Verification items for the finished model (mm, model axes). Face numbers are marked on the shaded views. A direction names the side the tool comes from. Coordinates: 2 decimals unless noted, no trailing zeros. Write each loop counter-clockwise with the first axis right and the second up, starting at its lowest first coordinate (ties: lowest second). Pieces come first, ordered by that corner, then holes. Notation, with made-up numbers: (61.5, -12) -> (68.5, -12) arc R36 cw to (68.5, 22) -> close; hole circle Ø3 at (1, 9). An arc over 180 degrees is marked (long way). Use CSV: the item, a comma, the result in double quotes.
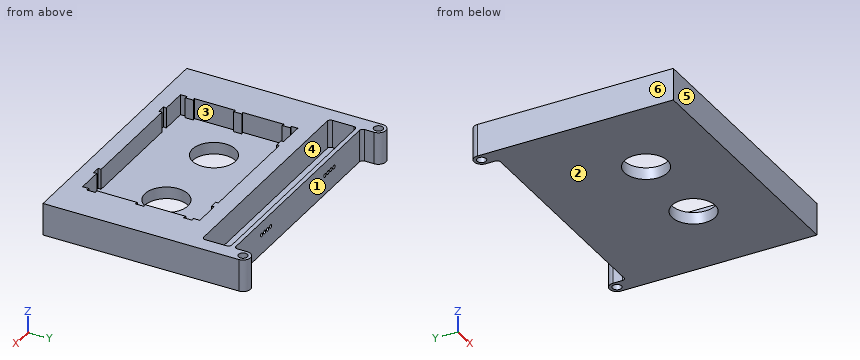
```python
from build123d import *

# Parameters (mm, degrees)
PAD001_DEPTH    = 9.5
SKETCH_R        = 2.1
PAD_DEPTH       = 15
POCKET_DEPTH    = 13
SKETCH003_R     = 10
POCKET001_DEPTH = 5.501
SKETCH004_R     = 0.85
POCKET002_DEPTH = 2


with BuildPart() as obj1:
    # Sketch002 → Pad001 (new body)
    with BuildSketch(Plane.XY):
        Polygon((-41.25, 27.25), (-29.15, 27.25), (-29.4, 26.05), (-25.6, 26.05), (-25.85, 27.25), (25.85, 27.25), (25.6, 26.05), (29.4, 26.05), (29.15, 27.25), (41.25, 27.25), (41.25, 24.25), (42.65, 24.5), (42.65, 20.5), (41.25, 20.75), (41.25, 1.75), (42.65, 2), (42.65, -2), (41.25, -1.75), (41.25, -20.75), (42.65, -20.5), (42.65, -24.5), (41.25, -24.25), (41.25, -27.25), (29.25, -27.25), (29.5, -28.65), (25.5, -28.65), (25.75, -27.25), (-25.75, -27.25), (-25.5, -28.65), (-29.5, -28.65), (-29.25, -27.25), (-41.25, -27.25), (-41.25, -24.15), (-40.05, -24.4), (-40.05, -20.6), (-41.25, -20.85), (-41.25, -1.65), (-40.05, -1.9), (-40.05, 1.9), (-41.25, 1.65), (-41.25, 20.85), (-40.05, 20.6), (-40.05, 24.4), (-41.25, 24.15), align=None)
    extrude(amount=-PAD001_DEPTH)


with BuildPart() as body:
    # Sketch → Pad (new body)
    with BuildSketch(Plane.XY):
        with BuildLine():
            Line((-52, 50), (52, 50))
            ThreePointArc((52, 50), (53.06066, 50.43934), (53.5, 51.5))
            Line((53.5, 51.5), (53.5, 56))
            ThreePointArc((60.5, 56), (57, 59.5), (53.5, 56))
            Line((60.5, 56), (60.5, -35))
            Line((60.5, -35), (-60.5, -35))
            Line((-60.5, 56), (-60.5, -35))
            ThreePointArc((-53.5, 56), (-57, 59.5), (-60.5, 56))
            Line((-53.5, 51.5), (-53.5, 56))
            ThreePointArc((-53.5, 51.5), (-53.06066, 50.43934), (-52, 50))
        make_face()
        with Locations((-57, 56)):
            Circle(SKETCH_R, mode=Mode.SUBTRACT)
        with Locations((57, 56)):
            Circle(SKETCH_R, mode=Mode.SUBTRACT)
    extrude(amount=-PAD_DEPTH)

    # Sketch001 (on Face13 of Pad) → Pocket (cut)
    with BuildSketch(Plane.XY):
        with BuildLine():
            Line((-52, 48), (52, 48))
            ThreePointArc((53.5, 46.5), (53.06066, 47.56066), (52, 48))
            Line((53.5, 46.5), (53.5, 36.5))
            ThreePointArc((52, 35), (53.06066, 35.43934), (53.5, 36.5))
            Line((52, 35), (-52, 35))
            ThreePointArc((-53.5, 36.5), (-53.06066, 35.43934), (-52, 35))
            Line((-53.5, 36.5), (-53.5, 46.5))
            ThreePointArc((-52, 48), (-53.06066, 47.56066), (-53.5, 46.5))
        make_face()
    extrude(amount=-POCKET_DEPTH, mode=Mode.SUBTRACT)

    # Boolean: cut obj1
    add(obj1.part, mode=Mode.SUBTRACT)

    # Sketch003 (on Face68 of Boolean) → Pocket001 (cut, through all)
    with BuildSketch(Plane.XY.offset(-9.5)):
        with Locations((-20, 0)):
            Circle(SKETCH003_R)
        with Locations((20, 0)):
            Circle(SKETCH003_R)
    extrude(amount=-POCKET001_DEPTH, mode=Mode.SUBTRACT)

    # Sketch004 (on Face3 of Pocket001) → Pocket002 (cut)
    with BuildSketch(Plane(origin=(0, 50, 0), x_dir=(-1, 0, 0), z_dir=(0, 1, 0))):
        with Locations((-30.48, -6)):
            Circle(SKETCH004_R)
        with Locations((-27.94, -6)):
            Circle(SKETCH004_R)
        with Locations((-25.4, -6)):
            Circle(SKETCH004_R)
        with Locations((-22.86, -6)):
            Circle(SKETCH004_R)
        with Locations((22.86, -6)):
            Circle(SKETCH004_R)
        with Locations((25.4, -6)):
            Circle(SKETCH004_R)
        with Locations((27.94, -6)):
            Circle(SKETCH004_R)
        with Locations((30.48, -6)):
            Circle(SKETCH004_R)
    extrude(amount=-POCKET002_DEPTH, mode=Mode.SUBTRACT)


solid = body.part
```
1) Cross-section at B-B (y = 6). Record the boundary of the cut face in (x, z), plus the area to 3 significant figures.
Return value:
outline,"(-60.5, -15) -> (-28, -15) -> (-28, -9.5) -> (-41.25, -9.5) -> (-41.25, 0) -> (-60.5, 0) -> close; (-12, -15) -> (12, -15) -> (12, -9.5) -> (-12, -9.5) -> close; (28, -15) -> (60.5, -15) -> (60.5, 0) -> (41.25, 0) -> (41.25, -9.5) -> (28, -9.5) -> close"
area,"855 mm2"
2) Gauge pin test, flat ends, axial feed: pin 1 (2 mm diameter, centred on x = -1.5, y = -25, fed in from +Z); pin 2 (4 mm diameter, centred on x = -7.5, y = 42, fed in from +Z); pin 3 (5 mm diameter, centred on x = -34, z = -3, fed in from +Y); pin 4 (1 mm diameter, centred on x = 20, y = 8, fed in from +Z). Record the tip position at first contact, or that the pin passes through.
Return value:
pin 1,"z = -9.5"
pin 2,"z = -13"
pin 3,"y = 50"
pin 4,"through"
3) Mould release check, pull along X, two halves, no side actions. Record for the marked faces 4, 5 and 6: released by +X, released by -X, zero draft, split by the parting line, or undercut.
Return value:
face 4,"undercut"
face 5,"zero draft"
face 6,"released by -X"
4) Cross-section at C-C (y = 39). Record the boundary of the cut face in (x, z), plus the area to 3 significant figures.
Return value:
outline,"(-60.5, -15) -> (60.5, -15) -> (60.5, 0) -> (53.5, 0) -> (53.5, -13) -> (-53.5, -13) -> (-53.5, 0) -> (-60.5, 0) -> close"
area,"424 mm2"
5) Cross-section at A-A (x = -57). Record the boundary of the cut face in (y, z), plus the area to 3 significant figures.
Return value:
outline,"(-35, -15) -> (53.9, -15) -> (53.9, 0) -> (-35, 0) -> close; (58.1, -15) -> (59.5, -15) -> (59.5, 0) -> (58.1, 0) -> close"
area,"1,350 mm2"
6) Cross-section at D-D (x = -6.5). Record the boundary of the cut face in (y, z), plus the area to 3 significant figures.
Return value:
outline,"(-35, -15) -> (50, -15) -> (50, 0) -> (48, 0) -> (48, -13) -> (35, -13) -> (35, 0) -> (27.25, 0) -> (27.25, -9.5) -> (-27.25, -9.5) -> (-27.25, 0) -> (-35, 0) -> close"
area,"588 mm2"
7) Set-up check for the marked faces 1, 2 and 3: record each of +Z, -Z, +X, -X, +Y, -Y from which the full face is reachable in a straight line by a thin tool's end or side.
Return value:
face 1,"+Z, -Z, +Y"
face 2,"-Z, +X, -X, +Y, -Y"
face 3,"+Z"
8) Scan lines: L1, parallel to Y at x = -9, z = -6.25; L2, parallel to Y at x = 20, z = -11.65; L3, parallel to Y at x = -19.5, z = -14.5. Record each from-to range of solid material in increasing order.
Return value:
L1,"-35 to -27.25, 27.25 to 35, 48 to 50"
L2,"-35 to -10, 10 to 35, 48 to 50"
L3,"-35 to -9.99, 9.99 to 50"
